from build123d import *

# Parameters (mm, degrees)
F0_R     = 63.5
F1_DEPTH = 19.05
F2_R     = 2.54
F3_R     = 2.54


with BuildPart() as f1:
    # F0 (on Right) → F1 (new body)
    with BuildSketch(Plane.YZ):
        Circle(F0_R)
    extrude(amount=F1_DEPTH)

    # F2
    f2_edges = [f1.edges().sort_by_distance(p)[0] for p in [
        (19.05, -63.5, 0),
    ]]
    fillet(f2_edges, radius=F2_R)

    # F3
    f3_edges = [f1.edges().sort_by_distance(p)[0] for p in [
        (0, -63.5, 0),
    ]]
    fillet(f3_edges, radius=F3_R)


solid = f1.part
The model under review builds one solid part; all positions refer to its coordinate system, in mm. Round coordinates to 2 decimals unless told otherwise and drop trailing zeros. Loops run counter-clockwise (first coordinate to the right, second up) from the corner with the lowest first, then second, coordinate; pieces in that order, holes last. Notation, with made-up numbers: (81.25, -5.75) -> (88.25, -5.75) arc R27 ccw to (88.25, 15.25) -> close; hole circle Ø6 at (-20, 29). An arc over 180 degrees is marked (long way). Return JSON: item names as keys, results as strings.
(1) For pin 1 (1 mm diameter, centred on x = 6.5, z = 39, fed in from +Y); pin 2 (3 mm diameter, centred on x = 3, z = 41, fed in from +Y); pin 3 (3 mm diameter, centred on x = 4, y = -38, fed in from -Z), all flat-tipped, find the tip position at first contact; note any pin that passes through.
Solved:
{"pin 1": "y = 50.5", "pin 2": "y = 49.72", "pin 3": "z = -51.96"}
(2) For line 1 (Z direction, x = 10, y = -12); line 2 (Z direction, x = 17.5, y = -56.5); line 3 (Y direction, x = 13.5, z = 45.5), list the stretches that pass through material, from the lowest coordinate up.
Solved:
{"line 1": "-62.36 to 62.36", "line 2": "-28.54 to 28.54", "line 3": "-44.29 to 44.29"}
(3) Add section A-A on x = 14.5. Write out the cut boundary in (y, z), plus the area to 3 significant figures.
Solved:
{"outline": "circle Ø127 at (0, 0)", "area": "12,700 mm2"}
